Can you work these out from the model? Positions are in its coordinate system, mm. Face numbers are marked on the shaded views. A direction names the side the tool comes from. Give positions to 0.01 mm unless a question says otherwise; leave off trailing zeros. Loops run counter-clockwise (first coordinate to the right, second up) from the corner with the lowest first, then second, coordinate; pieces in that order, holes last. Notation, with made-up numbers: (28, 67.5) - (41, 67.5) arc R20 ccw to (41, 88.5) - close; hole circle Ø1 at (84, -35). An arc over 180 degrees is marked (long way). Answer in a Markdown table with one row per item.
from build123d import *

# Parameters (mm, degrees)
AUFSATZ_LINEAR_AUSTRAGEN1_DEPTH = 10
SKIZZE2_R                       = 1.15
SCHNITT_LINEAR_AUSTRAGEN1_DEPTH = 11
SKIZZE3_R                       = 2.05
SCHNITT_LINEAR_AUSTRAGEN2_DEPTH = 2
SCHNITT_LINEAR_AUSTRAGEN3_DEPTH = 52.7
SCHNITT_LINEAR_START            = 1
SKIZZE5_R                       = 2.05
SCHNITT_LINEAR_AUSTRAGEN4_DEPTH = 10.0000001


with BuildPart() as part:
    # Skizze1 → Aufsatz-Linear austragen1 (new body)
    with BuildSketch(Plane.XY):
        Polygon((53.35, 39.925098055), (1.65, 39.925098055), (1.65, 46.925098055), (1.65, 55), (7, 55), (7, 60), (12, 65), (38.45220836, 65), (41, 58), (53.35, 58), (53.35, 46.925098055), align=None)
    extrude(amount=AUFSATZ_LINEAR_AUSTRAGEN1_DEPTH)

    # Skizze2 → Schnitt-Linear austragen1 (cut, through all)
    with BuildSketch(Plane.XY.offset(10)):
        with Locations((20, 43.425098055)):
            Circle(SKIZZE2_R)
    extrude(amount=-SCHNITT_LINEAR_AUSTRAGEN1_DEPTH, mode=Mode.SUBTRACT)

    # Skizze3 → Schnitt-Linear austragen2 (cut)
    with BuildSketch(Plane.XY.offset(10)):
        with Locations((20, 43.425098055)):
            Circle(SKIZZE3_R)
    extrude(amount=-SCHNITT_LINEAR_AUSTRAGEN2_DEPTH, mode=Mode.SUBTRACT)

    # Skizze4 → Schnitt-Linear austragen3 (cut, through all)
    with BuildSketch(Plane(origin=(53.35, 0, 0), x_dir=(0, 0, -1), z_dir=(1, 0, 0))):
        with BuildLine():
            Line((-10, 65), (-48.166713837, 39.925098055))
            Line((-48.166713837, 39.925098055), (-2.5, 39.925098055))
            ThreePointArc((-2.5, 39.925098055), (-4.415158713, 53.011357142), (-10, 65))
        make_face()
    extrude(amount=-SCHNITT_LINEAR_AUSTRAGEN3_DEPTH, mode=Mode.SUBTRACT)

    # Skizze5 → Schnitt-Linear austragen4 (cut, through all)
    with BuildSketch(Plane.XY.offset(SCHNITT_LINEAR_START)):
        with Locations((20, 43.425098055)):
            Circle(SKIZZE5_R)
    extrude(amount=SCHNITT_LINEAR_AUSTRAGEN4_DEPTH, mode=Mode.SUBTRACT)


solid = part.part
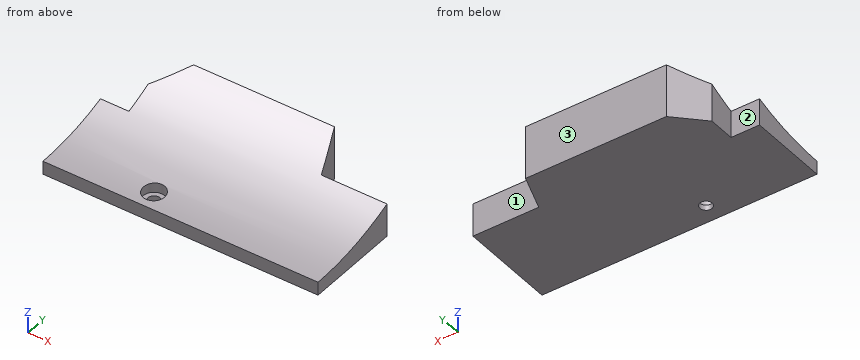
Q1. Imagine slicing it at B-B, the plane z = 1.75. Write out the boundary of the cut face in (x, y).
Checked values:
| item | result |
|---|---|
| outline | (1.65, 39.93) - (53.35, 39.93) - (53.35, 58) - (41, 58) - (38.45, 65) - (12, 65) - (7, 60) - (7, 55) - (1.65, 55) - close; hole circle Ø4.1 at (20, 43.43) |
Q2. If I drill on line 1 (Y direction, x = 20, z = 2.4); line 2 (Y direction, x = 20, z = 0.4); line 3 (Z direction, x = 17, y = 45.5), over which ranges is the centre line in solid material (lowest first)? Write a range as [from, to].
Checked values:
| item | result |
|---|---|
| line 1 | y = [39.93, 41.38], [45.48, 65] |
| line 2 | y = [39.93, 42.28], [44.58, 65] |
| line 3 | z = [0, 2.84] |
Q3. On a 3-axis mill with a long thin cutter (end or side, diameter ignored), from which of +Z, -Z, +X, -X, +Y, -Y can I reach the whole of each face in a straight line? I mean the marked faces 1, 2 and 3. Say none if no direction works.
Checked values:
| item | result |
|---|---|
| face 1 | +Z, -Z, +X, +Y |
| face 2 | +Z, -Z, -X, +Y |
| face 3 | +Z, -Z, +X, -X, +Y |
Q4. Imagine slicing it at D-D, the plane y = 49.75. Write out the boundary of the cut face in (x, z), and give its area (3 significant figures).
Checked values:
| item | result |
|---|---|
| outline | (1.65, 0) - (53.35, 0) - (53.35, 3.57) - (1.65, 3.57) - close |
| area | 185 mm² |
Q5. Imagine slicing it at C-C, the plane x = 5. Write out the boundary of the cut face in (y, z).
Checked values:
| item | result |
|---|---|
| outline | (39.93, 0) - (55, 0) - (55, 5.06) arc R45.67 cw to (39.93, 2.5) - close |
Q6. For pin 1 (1.5 mm diameter, centred on x = 12.5, y = 51, fed in from -Z); pin 2 (1.5 mm diameter, centred on y = 57.5, z = 2.5, fed in from -X); pin 3 (10 mm diameter, centred on x = 43, y = 56, fed in from +Z); pin 4 (2 mm diameter, centred on x = 34.5, z = 8, fed in from -Y), each with a flat end and sliding along its axis, tell me the tip position at first contact or that it passes through.
Checked values:
| item | result |
|---|---|
| pin 1 | stops at z = 0 |
| pin 2 | stops at x = 7 |
| pin 3 | stops at z = 7.22 |
| pin 4 | stops at y = 59.69 |
Q7. Imagine slicing it at A-A, the plane x = 20. Write out the boundary of the cut face in (y, z).
Checked values:
| item | result |
|---|---|
| outline | (39.93, 0) - (42.28, 0) - (42.28, 1) - (41.38, 1) - (41.38, 2.52) arc R45.67 cw to (39.93, 2.5) - close; (44.58, 0) - (65, 0) - (65, 10) arc R45.67 cw to (45.48, 2.84) - (45.48, 1) - (44.58, 1) - close |
